Input: part model. Units: mm. Frame: model coordinates. A direction names the side the tool comes from. Round coordinates to 2 decimals unless told otherwise and drop trailing zeros. Loops run counter-clockwise (first coordinate to the right, second up) from the corner with the lowest first, then second, coordinate; pieces in that order, holes last.
1) Section B-B, the plane z = 2. Return loops of the section in (x, y), and give its area (3 significant figures).
2) Access query for faces 1 (the face through (67.77, 14.78, 4.52)), 2 (the face through (-9.976, -9, 5)), 3 (the face through (-26.476, 6, 5)), 4 (the face through (19, 28.625, 5)). Directions: +Z, -Z, +X, -X, +Y, -Y. A direction counts if a zero-diameter tool reaches every point of the face in a straight line with its end or side. Return the directions, or none.
3) Draft query along Y for faces 5 (the face through (19, -24.375, 5)), 6 (the face through (-27.721, -8.383, 4.239)), 7 (the face through (85.024, 2, 5)), 8 (the face through (-9.976, 14, 5)). Return one class per face: pulls with the +Y half, pulls with the -Y half, needs draft (parallel to the pull), parting line crosses it, or undercut.
4) Ray query, line 1 along X through (y, z) = (26, 4.75); line 2 along X through (y, z) = (5.5, 9); line 3 along Y through (x, z) = (57, 2). Return the intervals inside material, ascending.
5) First-contact query: pin 1 (1.5 mm diameter, centred on x = -4.98, z = 5, fed in from -Y); pin 2 (0.8 mm diameter, centred on y = -9.5, z = 4.5, fed in from -X). Flat tips, straight axial feed; report the tip coordinate or a pass-through.
6) Section A-A, the plane y = 2. Return loops of the section in (x, z).
from build123d import *

# Parameters (mm, degrees)
F0_W     = 130
F0_H     = 53
F1_DEPTH = 10
F2_R     = 1.25
F5_DEPTH = 35
F3_R     = 1.25
F6_DEPTH = 53
F4_R     = 1.25
F7_DEPTH = 35
F9_DEPTH = 10


with BuildPart() as f1:
    # F0 (on Top) → F1 (new body)
    with BuildSketch(Plane.XY):
        with Locations((20.023906, 2.124549)):
            Rectangle(F0_W, F0_H)
    extrude(amount=F1_DEPTH)

    # F2 (on face) → F5 (cut)
    with BuildSketch(Plane.YZ.offset(85.023906)):
        with Locations((-9.375451, 5)):
            Circle(F2_R)
        with Locations((13.624549, 5)):
            Circle(F2_R)
    extrude(amount=-F5_DEPTH, mode=Mode.SUBTRACT)

    # F3 (on face) → F6 (cut, through all)
    with BuildSketch(Plane.XZ.offset(24.375451)):
        with Locations((-4.976094, 5)):
            Circle(F3_R)
        with Locations((45.023906, 5)):
            Circle(F3_R)
    extrude(amount=-F6_DEPTH, mode=Mode.SUBTRACT)

    # F4 (on face) → F7 (cut)
    with BuildSketch(Plane(origin=(-44.976094, 0, 0), x_dir=(0, -1, 0), z_dir=(-1, 0, 0))):
        with Locations((-13.624549, 5)):
            Circle(F4_R)
        with Locations((9.375451, 5)):
            Circle(F4_R)
    extrude(amount=-F7_DEPTH, mode=Mode.SUBTRACT)

    # F8 (on face) → F9 (cut, through all)
    with BuildSketch(Plane.XY.offset(10)):
        with BuildLine():
            Line((66.523906, -1.249315), (66.523906, 12.498412))
            ThreePointArc((66.523906, 12.498412), (56.023906, 5.624549), (66.523906, -1.249315))
        make_face()
        with BuildLine():
            ThreePointArc((-26.476094, -1.249315), (-19.368175, -0.650401), (-15.976094, 5.624549))
            ThreePointArc((-15.976094, 5.624549), (-19.368175, 11.899499), (-26.476094, 12.498412))
            Line((-26.476094, 12.498412), (-26.476094, -1.249315))
        make_face()
    extrude(amount=-F9_DEPTH, mode=Mode.SUBTRACT)


solid = f1.part
Final values:
1. outline: (-44.98, -24.38) - (85.02, -24.38) - (85.02, 28.62) - (-44.98, 28.62) - close; hole (-26.48, -1.25) arc R7.5 ccw to (-15.98, 5.62) arc R7.5 ccw to (-26.48, 12.5) - close; hole (66.52, -1.25) - (66.52, 12.5) arc R7.5 ccw (long way) to start
1. area: 6,630 mm2
2. face 1: +X
2. face 2: -X
2. face 3: +Z, -Z
2. face 4: +Z, -Z, +X, -X, +Y
3. face 5: pulls with the -Y half
3. face 6: undercut
3. face 7: needs draft
3. face 8: undercut
4. line 1: x = -44.98 to -6.2, -3.75 to 43.8, 46.25 to 85.02
4. line 2: x = -44.98 to -26.48, -15.98 to 56.02, 66.52 to 85.02
4. line 3: y = -24.38 to 1.92, 9.32 to 28.62
5. pin 1: passes through
5. pin 2: stops at x = -9.98
6. outline: (-44.98, 0) - (-26.48, 0) - (-26.48, 10) - (-44.98, 10) - close; (-16.91, 0) - (56.96, 0) - (56.96, 10) - (-16.91, 10) - close; (66.52, 0) - (85.02, 0) - (85.02, 10) - (66.52, 10) - close; hole circle Ø2.5 at (-4.98, 5); hole circle Ø2.5 at (45.02, 5)
